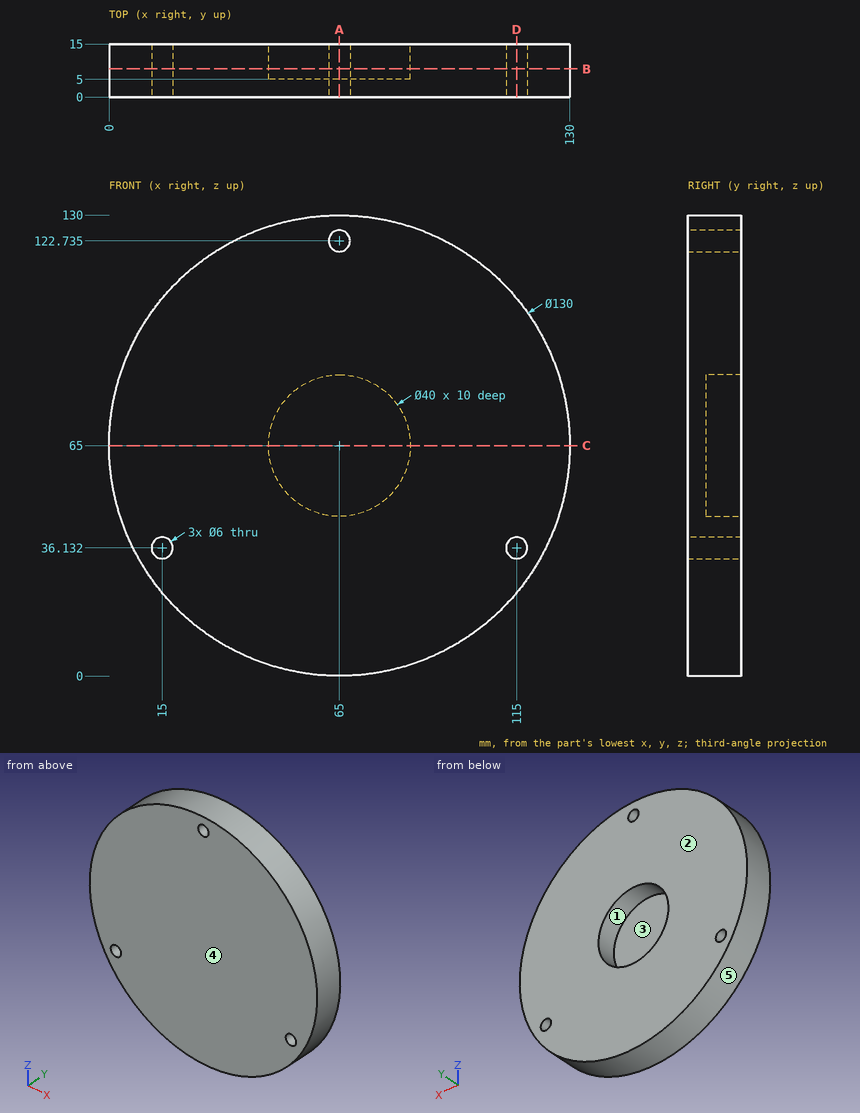
Geometry check sheet. Reference: drawing and pictorial views, mm from the part's lowest x, y, z. A direction names the side the tool comes from. Coordinates: 2 decimals unless noted, no trailing zeros. Order: outer loops, then holes, each group sorted by start corner. A loop starts at its lowest first (then second) coordinate and runs counter-clockwise, first axis right, second up. Notation, with made-up numbers: (73.25, 64.5) -> (94.25, 64.5) arc R14 ccw to (94.25, 70.5) -> close; hole circle Ø11 at (80, 48). An arc over 180 degrees is marked (long way). Put each result on its own line as item: value. Start each with the question number.
1) Tool access check on the marked faces 1 and 2. Record the directions out of +Z, -Z, +X, -X, +Y, -Y that give a thin tool (end or side, any length) a straight path to the whole face; none if there is none.
2) Cross-section at B-B (y = 8). Enter the section's corners in (x, z) (1 decimal), plus the area to 3 significant figures.
3) Release check for a two-part mould opening along X. For the marked faces 3, 4 and 5 record: pulls with the +X half, pulls with the -X half, needs draft (parallel to the pull), parting line crosses it, or undercut.
4) Cross-section at D-D (x = 115). Enter the section's corners in (y, z).
5) Go/stop test with flat-tipped pins: pin 1 (1.5 mm diameter, centred on x = 107, y = 6, fed in from +Z) (1 decimal); pin 2 (4 mm diameter, centred on y = 2.5, z = 45, fed in from -X); pin 3 (5.5 mm diameter, centred on x = 65, z = 122.74, fed in from +Y); pin 4 (1.5 mm diameter, centred on x = 33, y = 7, fed in from -Z) (1 decimal). Record where each tip stops, or that it passes through.
6) Material ranges on L1, parallel to X at y = 10.5, z = 65; L2, parallel to Z at x = 13.5, y = 13.75 (1 decimal); L3, parallel to Z at x = 63.5, y = 8.25 (1 decimal), recorded low to high.
7) Cross-section at C-C (z = 65). Enter the section's corners in (x, y).
8) Cross-section at A-A (x = 65). Enter the section's corners in (y, z) (1 decimal).
Geometry check:
1. face 1: +Y
1. face 2: +Z, -Z, +X, -X, +Y
2. outline: circle Ø130 at (65, 65); hole circle Ø6 at (15, 36.1); hole circle Ø40 at (65, 65); hole circle Ø6 at (65, 122.7); hole circle Ø6 at (115, 36.1)
2. area: 11,900 mm^2
3. face 3: undercut
3. face 4: needs draft
3. face 5: parting line crosses it
4. outline: (0, 23.47) -> (15, 23.47) -> (15, 33.13) -> (0, 33.13) -> close; (0, 39.13) -> (15, 39.13) -> (15, 106.53) -> (0, 106.53) -> close
5. pin 1: stops at z = 115.2
5. pin 2: stops at x = 2.54
5. pin 3: passes through
5. pin 4: stops at z = 8
6. L1: x = 0 to 45, 85 to 130
6. L2: z = 25.3 to 33.5, 38.7 to 104.7
6. L3: z = 0 to 45.1, 84.9 to 120.1, 125.3 to 130
7. outline: (0, 0) -> (130, 0) -> (130, 15) -> (85, 15) -> (85, 5) -> (45, 5) -> (45, 15) -> (0, 15) -> close
8. outline: (0, 0) -> (15, 0) -> (15, 45) -> (5, 45) -> (5, 85) -> (15, 85) -> (15, 119.7) -> (0, 119.7) -> close; (0, 125.7) -> (15, 125.7) -> (15, 130) -> (0, 130) -> close
